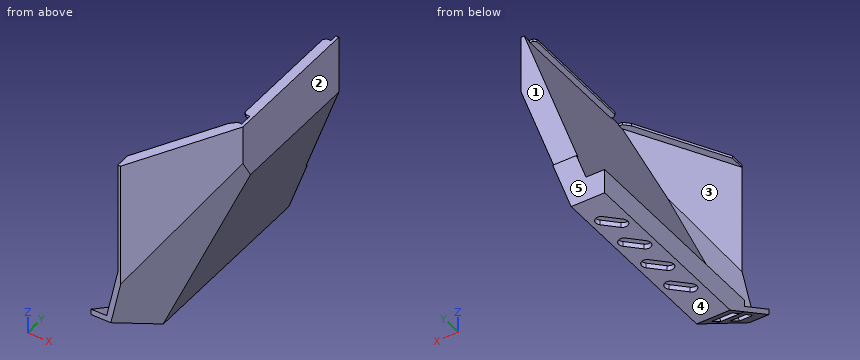
from build123d import *
from OCP.BRepFilletAPI import BRepFilletAPI_MakeChamfer

# Parameters (mm, degrees)
BOSS_EXTRU_2_DEPTH            = 850
ESQUISSE2_W                   = 135.455554094
ESQUISSE2_H                   = 850
BOSS_EXTRU_4_DEPTH            = 100
ESQUISSE7_W                   = 615
ESQUISSE7_H                   = 10
ENL_V_MAT_EXTRU_5_DEPTH       = 1260.158602645
ENL_V_MAT_EXTRU_6_DEPTH       = 1237.105055174
CHANFREIN1_SIZE               = 40
CHANFREIN1_SIZE2              = 104.203562588
CHANFREIN2_SIZE               = 50
CHANFREIN2_SIZE2              = 86.602540378
CHANFREIN3_SIZE               = 250
CHANFREIN3_SIZE2              = 81.394715296
ENL_V_MAT_EXTRU_9_DEPTH       = 20
BOSS_EXTRU_5_DEPTH            = 20
BOSS_EXTRU_6_DEPTH            = 20
BOSS_EXTRU_7_DEPTH            = 20
BOSS_EXTRU_8_REACH            = 1235.856
BOSS_EXTRU_14_REACH           = 1078.841
ENL_V_MAT_EXTRU_11_DEPTH      = 1231.067968745
ENL_V_MAT_EXTRU_11_DEPTH_BACK = 1231.067968745
ESQUISSE20_W                  = 36.798592216
ESQUISSE20_H                  = 35.835276246
ENL_V_MAT_EXTRU_10_DEPTH      = 1231.067968745
ENL_V_MAT_EXTRU_10_DEPTH_BACK = 1231.067968745
BOSS_EXTRU_15_DEPTH           = 10
ENL_V_MAT_EXTRU_12_DEPTH      = 1231.067968745
BOSS_EXTRU_17_DEPTH           = 10
ENL_V_MAT_EXTRU_13_DEPTH      = 10
CHANFREIN6_SIZE               = 10
CHANFREIN6_SIZE2              = 25.739216822
ENL_V_MAT_EXTRU_7_DEPTH       = 20
ESQUISSE28_W                  = 50.106872135
ESQUISSE28_H                  = 235.71179502
ENL_V_MAT_EXTRU_15_DEPTH      = 1231.067968745


with BuildPart() as part:
    # Esquisse1 → Boss.-Extru.2 (new body)
    with BuildSketch(Plane(origin=(0, 0, 0), x_dir=(1, 0, 0), z_dir=(0, 1, 0))):
        Polygon((0, 0), (95.455554093, 0), (-196.119788372, 825), (-291.575342466, 825), align=None)
    extrude(amount=BOSS_EXTRU_2_DEPTH)

    # Esquisse2 → Boss.-Extru.4 (add)
    with BuildSketch(Plane(origin=(0, 0, -825), x_dir=(-1, 0, 0), z_dir=(0, 0, -1))):
        with Locations((263.847565419, 425)):
            Rectangle(ESQUISSE2_W, ESQUISSE2_H)
    extrude(amount=-BOSS_EXTRU_4_DEPTH)

    # Esquisse7 → Enlèv. mat.-Extru.5 (cut, through all)
    with BuildSketch(Plane.ZY.offset(331.575342466)):
        with Locations((-307.5, 845)):
            Rectangle(ESQUISSE7_W, ESQUISSE7_H)
    extrude(amount=-ENL_V_MAT_EXTRU_5_DEPTH, mode=Mode.SUBTRACT)

    # Esquisse8 → Enlèv. mat.-Extru.6 (cut, through all)
    with BuildSketch(Plane(origin=(84.856246207, 0, -29.990289755), x_dir=(-0.3332254417270876, 0, -0.9428471800805194), z_dir=(0.9428471800805194, 0, -0.3332254417270876))):
        Polygon((-31.808219178, 280), (768.947519086, 0), (-31.808219178, 0), align=None)
    extrude(amount=-ENL_V_MAT_EXTRU_6_DEPTH, mode=Mode.SUBTRACT)

    # Chanfrein1
    chanfrein1_edges = [part.edges().sort_by_distance(p)[0] for p in [
        (-37.960538206, 140, -377.495144878),
    ]]
    chanfrein1_side = [part.faces().sort_by_distance(p)[0] for p in [
        (-82.734004125, 137.238189401, -370.048215647),
    ]]
    chamfer(chanfrein1_edges, length=CHANFREIN1_SIZE, length2=CHANFREIN1_SIZE2, reference=chanfrein1_side[0])

    # Chanfrein2
    chanfrein2_edges = [part.edges().sort_by_distance(p)[0] for p in [
        (-279.375357295, 0, -825),
    ]]
    chanfrein2_side = [part.faces().sort_by_distance(p)[0] for p in [
        (-275.691218494, 0, -775.06397156),
    ]]
    chamfer(chanfrein2_edges, length=CHANFREIN2_SIZE, length2=CHANFREIN2_SIZE2, reference=chanfrein2_side[0])

    # Chanfrein3
    chanfrein3_edges = [part.edges().sort_by_distance(p)[0] for p in [
        (95.455554093, 615.195164523, 0),
    ]]
    chanfrein3_side = [part.faces().sort_by_distance(p)[0] for p in [
        (-63.074276605, 533.547742021, -448.553396936),
    ]]
    chamfer(chanfrein3_edges, length=CHANFREIN3_SIZE, length2=CHANFREIN3_SIZE2, reference=chanfrein3_side[0])

    # Esquisse11 → Enlèv. mat.-Extru.9 (cut)
    with BuildSketch(Plane(origin=(0, 0, -825), x_dir=(-1, 0, 0), z_dir=(0, 0, -1))):
        with BuildLine():
            Line((273.165439889, 663.862320377), (222.709885796, 714.31787447))
            ThreePointArc((222.709885796, 714.31787447), (222.709885796, 746.137679623), (254.529690949, 746.137679623))
            Line((254.529690949, 746.137679623), (304.985245042, 695.68212553))
            ThreePointArc((304.985245042, 695.68212553), (304.985245042, 663.862320377), (273.165439889, 663.862320377))
        make_face()
        with BuildLine():
            Line((273.165439889, 523.862320377), (222.709885796, 574.31787447))
            ThreePointArc((222.709885796, 574.31787447), (222.709885796, 606.137679623), (254.529690949, 606.137679623))
            Line((254.529690949, 606.137679623), (304.985245042, 555.68212553))
            ThreePointArc((304.985245042, 555.68212553), (304.985245042, 523.862320377), (273.165439889, 523.862320377))
        make_face()
        with BuildLine():
            Line((273.165439889, 383.862320377), (222.709885796, 434.31787447))
            ThreePointArc((222.709885796, 434.31787447), (222.709885796, 466.137679623), (254.529690949, 466.137679623))
            Line((254.529690949, 466.137679623), (304.985245042, 415.68212553))
            ThreePointArc((304.985245042, 415.68212553), (304.985245042, 383.862320377), (273.165439889, 383.862320377))
        make_face()
        with BuildLine():
            Line((273.165439889, 243.862320377), (222.709885796, 294.31787447))
            ThreePointArc((222.709885796, 294.31787447), (222.709885796, 326.137679623), (254.529690949, 326.137679623))
            Line((254.529690949, 326.137679623), (304.985245042, 275.68212553))
            ThreePointArc((304.985245042, 275.68212553), (304.985245042, 243.862320377), (273.165439889, 243.862320377))
        make_face()
    extrude(amount=-ENL_V_MAT_EXTRU_9_DEPTH, mode=Mode.SUBTRACT)

    # Esquisse12 → Boss.-Extru.5 (add)
    with BuildSketch(Plane(origin=(-40.719657631, 14.978452192, 8.836336942), x_dir=(-0.1789623557208966, 0.09138543974154965, -0.9796025605509977), z_dir=(0.9196400605905344, -0.33828341108028354, -0.19956576045235425))):
        Polygon((758.2962151, -87.760898196), (129.510578012, 220.360980406), (128.5939647, -274.639019594), (551.387234827, -304.990440115), align=None)
    extrude(amount=-BOSS_EXTRU_5_DEPTH)

    # Esquisse13 → Boss.-Extru.6 (add)
    with BuildSketch(Plane(origin=(0, -335.584843966, -581.25), x_dir=(-1, 0, 0), z_dir=(0, -0.5000000000000013, -0.8660254037844379))):
        Polygon((331.575342466, 387.5), (216.325161863, 387.5), (331.575342466, -161.154885751), align=None)
    extrude(amount=-BOSS_EXTRU_6_DEPTH)

    # Esquisse14 → Boss.-Extru.7 (add)
    with BuildSketch(Plane(origin=(-40.719657631, 14.978452192, 8.836336942), x_dir=(0.18729623755068028, -0.06889566128781024, 0.9798844356632441), z_dir=(-0.9196400605905354, 0.33828341108028165, 0.19956576045235197))):
        Polygon((-558.543564559, -291.678140731), (-760.182954736, -69.548547185), (-765.904204326, -72.183872894), (-799.927326543, -74.681473645), (-671.74280044, -297.07939729), align=None)
    extrude(amount=BOSS_EXTRU_7_DEPTH)

    # Boss.-Extru.8: up to this face of the body (flat: up to its plane)
    boss_extru_8_end = Plane(part.part.faces().sort_by_distance((-164.532158793, -37.982859016, -371.724952169))[0])
    # Esquisse17 → Boss.-Extru.8 (add, up to the picked face)
    with BuildSketch(Plane(origin=(14.059914026, 0, -0.114027244), x_dir=(-0.008109828661301803, 0, -0.9999671147988239), z_dir=(0.999967114798824, 0, -0.008109828661301803)), mode=Mode.PRIVATE) as boss_extru_8_sk1:
        Polygon((0, 268.877630288), (0, -254.375489576), (124.880630316, -230.495880912), (112.743376241, 233.203159991), align=None)
    boss_extru_8_tool1 = split(extrude(boss_extru_8_sk1.sketch, amount=-BOSS_EXTRU_8_REACH, mode=Mode.PRIVATE), bisect_by=boss_extru_8_end, keep=Keep.BOTH, mode=Mode.PRIVATE)
    add(boss_extru_8_tool1.solids().sort_by(Axis((13.587491, -0.094835, -58.365221), (-0.999967114798824, 0, 0.008109828661301803)))[0])

    # Boss.-Extru.14: up to this face of the body (flat: up to its plane)
    boss_extru_14_end = Plane(part.part.faces().sort_by_distance((-146.671728248, -30.602018057, -301.931660273))[0])
    # Esquisse19 → Boss.-Extru.14 (add, up to the picked face)
    with BuildSketch(Plane(origin=(-27.916044034, 239.583966402, -78.987256375), x_dir=(-0.9939328490713287, -0.1044581087967751, 0.034438278754206304), z_dir=(0.1099885973042266, -0.9439555392983614, 0.31120804663599005)), mode=Mode.PRIVATE) as boss_extru_14_sk1:
        Polygon((-42.23311753, -84.700642173), (-41.849173409, -35.141174806), (202.602212611, 697.589071061), (229.71052108, 688.54527409), (-28.086448758, -84.187661354), align=None)
    boss_extru_14_tool1 = split(extrude(boss_extru_14_sk1.sketch, amount=BOSS_EXTRU_14_REACH, mode=Mode.PRIVATE), bisect_by=boss_extru_14_end, keep=Keep.BOTH, mode=Mode.PRIVATE)
    add(boss_extru_14_tool1.solids().sort_by(Axis((-116.11325, 133.026087, -371.027306), (0.1099885973042266, -0.9439555392983614, 0.31120804663599005)))[0])

    # Esquisse20 → Enlèv. mat.-Extru.11 (cut, two sides: drawn at the far end of the back side and taken through both)
    with BuildSketch(Plane(origin=(0, 0, 0), x_dir=(1, 0, 0), z_dir=(0, 1, 0)).offset(-ENL_V_MAT_EXTRU_11_DEPTH_BACK)):
        with Locations((-4.33845731, -17.917638123)):
            Rectangle(ESQUISSE20_W, ESQUISSE20_H)
    extrude(amount=ENL_V_MAT_EXTRU_11_DEPTH + ENL_V_MAT_EXTRU_11_DEPTH_BACK, mode=Mode.SUBTRACT)

    # Esquisse15 → Enlèv. mat.-Extru.10 (cut, two sides: drawn at the far end of the back side and taken through both)
    with BuildSketch(Plane.XY.offset(-ENL_V_MAT_EXTRU_10_DEPTH_BACK)):
        Polygon((-331.575342466, -190.149068971), (-331.575342466, -475.149068971), (14.059914026, -475.149068971), (14.059914026, -190.149068971), (55.846885337, -190.149068971), (55.846885337, 19.850931029), (55.846885337, 270.515982808), (14.060838798, 270.515982808), (14.060838798, 259.850931029), (-235.940085974, -190.149068971), align=None)
    extrude(amount=ENL_V_MAT_EXTRU_10_DEPTH + ENL_V_MAT_EXTRU_10_DEPTH_BACK, mode=Mode.SUBTRACT)

    # Esquisse21 → Boss.-Extru.15 (add)
    with BuildSketch(Plane(origin=(-99.569705588, 55.316707725, 0), x_dir=(0, 0, -1), z_dir=(0.8741565134833756, -0.4856443039247848, 0))):
        Polygon((321.424737861, -305.542159578), (543.068402305, -280.803005995), (155.773656423, 231.37758287), (0, 233.978950164), (0, 205.025992858), (0, -305.542159578), align=None)
    extrude(amount=-BOSS_EXTRU_15_DEPTH)

    # Esquisse23 → Enlèv. mat.-Extru.12 (cut, through all)
    with BuildSketch(Plane.XY):
        Polygon((-331.575342466, -190.149068971), (-331.575342466, -260.816411821), (-102.082537534, -260.816411821), (-102.082537534, -190.149068971), (-102.082537534, -148.149068971), (-331.575342466, -148.149068971), align=None)
    extrude(amount=-ENL_V_MAT_EXTRU_12_DEPTH, mode=Mode.SUBTRACT)

    # Esquisse26 → Boss.-Extru.17 (add)
    with BuildSketch(Plane.XY):
        Polygon((14.060838798, 810), (14.060838798, 317.576928865), (-25.939161202, 317.576928865), (-25.939161202, 810), (0, 810), (0, 840), (14.060838798, 840), align=None)
        Polygon((-25.939161202, 267.576928865), (14.060838798, 267.576928865), (12.797499589, 257.576928865), (-212.606666329, -148.149068971), (-224.046265355, -148.149068971), (-224.046265355, -89.014539546), align=None)
    extrude(amount=-BOSS_EXTRU_17_DEPTH)

    # Esquisse24 → Enlèv. mat.-Extru.13 (cut)
    with BuildSketch(Plane(origin=(14.059914026, 0, -0.114027244), x_dir=(-0.008109828661301803, 0, -0.9999671147988239), z_dir=(0.999967114798824, 0, -0.008109828661301803))):
        Polygon((-0.114030993, 259.850931029), (155.664748246, 257.576928865), (235.605515711, 302.972909907), (235.605515711, 840), (-0.114030993, 840), align=None)
    extrude(amount=ENL_V_MAT_EXTRU_13_DEPTH, mode=Mode.SUBTRACT)

    # Chanfrein6: one chamfer whose edges measure the first distance from different faces: ONE call of the kernel's chamfer builder (chamfer() names one face for all edges)
    chanfrein6_edges_1 = [part.edges().sort_by_distance(p)[0] for p in [
        (-25.939161202, 267.576928865, -5),
    ]]
    chanfrein6_side_1 = [part.faces().sort_by_distance(p)[0] for p in [
        (-13.831610998, 267.576928865, -4.878156509),
    ]]
    chanfrein6_edges_2 = [part.edges().sort_by_distance(p)[0] for p in [
        (-25.939161202, 810, -5),
        (-25.939161202, 317.576928865, -5),
    ]]
    chanfrein6 = BRepFilletAPI_MakeChamfer(part.part.solid().wrapped)
    for e in chanfrein6_edges_1:
        chanfrein6.Add(CHANFREIN6_SIZE, CHANFREIN6_SIZE2, e.wrapped, chanfrein6_side_1[0].wrapped)  # the first distance lies on this face
    for e in chanfrein6_edges_2:
        chanfrein6.Add(CHANFREIN6_SIZE, e.wrapped)
    add(Compound.cast(chanfrein6.Shape()), mode=Mode.REPLACE)

    # Esquisse9 → Enlèv. mat.-Extru.7 (cut)
    with BuildSketch(Plane(origin=(0, -335.584843966, -581.25), x_dir=(-1, 0, 0), z_dir=(0, -0.49999999999999656, -0.8660254037844407))):
        Polygon((311.575342466, 438.386921888), (226.072366588, 438.386921888), (236.575342466, 388.386921888), (311.575342466, 388.386921888), align=None)
        Polygon((311.575342466, 343.175811089), (246.072366588, 343.175811089), (256.575342466, 293.175811089), (311.575342466, 293.175811089), align=None)
    extrude(amount=-ENL_V_MAT_EXTRU_7_DEPTH, mode=Mode.SUBTRACT)

    # Esquisse28 → Enlèv. mat.-Extru.15 (cut, through all)
    with BuildSketch(Plane(origin=(0, 0, 0), x_dir=(1, 0, 0), z_dir=(0, 1, 0))):
        with Locations((37.20262973, 117.85589751)):
            Rectangle(ESQUISSE28_W, ESQUISSE28_H)
    extrude(amount=ENL_V_MAT_EXTRU_15_DEPTH, mode=Mode.SUBTRACT)


solid = part.part
The model under review builds one solid part; all positions refer to its coordinate system, in mm. Face numbers are marked on the shaded views. A direction names the side the tool comes from. Give positions to 0.01 mm unless a question says otherwise; leave off trailing zeros. Write each loop counter-clockwise with the first axis right and the second up, starting at its lowest first coordinate (ties: lowest second). Pieces come first, ordered by that corner, then holes.
1. Add section C-C, the plane x = -62. Write out the cut boundary in (y, z), plus the area to 3 significant figures.
2. For P1, Ø3, axis at y = -118.5, z = -3, coming from the -X side; P2, Ø6, axis at y = 343.5, z = -161, coming from the -X side; P3, Ø5, axis at x = -149.5, y = 846, coming from the +Z side, all flat-tipped, find the tip position at first contact; note any pin that passes through.
3. Add section D-D, the plane y = 168.5. Write out the cut boundary in (x, z).
4. Tool access review of the marked faces 1 and 2: name each direction out of +Z, -Z, +X, -X, +Y, -Y from which nothing blocks a thin tool from reaching the whole face with its end or side.
5. Wall thickness on L1, parallel to X at y = 389, z = -433; L2, parallel to X at y = -105.5, z = -559.5; L3, parallel to Y at x = -38.5, z = -157: over which ranges is each line inside the solid? List them lowest first.
6. Add section B-B, the plane z = -446. Write out the cut boundary in (x, y).
7. Draft analysis for pull direction Z (two halves, no side actions). For the marked faces 3, 4 and 5, state which applies: +Z half, -Z half, draft (parallel to the pull), parting line (faces both ways), or undercut.
8. Add section A-A, the plane y = 785. Write out the cut boundary in (x, z), plus the area to 3 significant figures.
Worked answers:
1. outline: (122.94, -272.24) - (225.16, -445.51) - (840, -445.51) - (840, -175.43) - (143.53, -175.43) - (143.53, -10) - (202.67, -10) - (202.67, 0) - (122.94, 0) - close
1. area: 189,000 mm2
2. P1: stops at x = -224.05
2. P2: stops at x = -57.96
2. P3: stops at z = -615
3. outline: (-331.58, -825) - (-196.12, -825) - (-116, -598.3) - (-36.69, -232.83) - (-36.69, 0) - (-80.98, 0) - (-80.98, -10) - (-48.13, -10) - (-48.13, -136.18) - (-256.23, -725) - (-331.58, -725) - close
4. face 1: +Z, +X, -X, +Y
4. face 2: +Z, -Z, +X, +Y, -Y
5. L1: x = -153.03 to -57.58
5. L2: x = -230.12 to -208.37
5. L3: y = 165.24 to 840
6. outline: (-224.05, -148.15) - (-212.61, -148.15) - (-173.6, -77.93) - (-62.17, 224.98) - (-62.17, 840) - (-157.63, 840) - (-157.63, 24.61) - (-215.55, -132.85) - close
7. face 3: undercut
7. face 4: -Z half
7. face 5: draft
8. outline: (-331.58, -825) - (-196.12, -825) - (12.15, -235.71) - (12.15, 0) - (-25.94, 0) - (-25.94, -10) - (-3.53, -10) - (-256.23, -725) - (-331.58, -725) - close
8. area: 74,900 mm2
